from build123d import *

# Parameters (mm, degrees)
SKETCH1_W           = 25.42
SKETCH1_H           = 25.42
BOSS_EXTRUDE5_DEPTH = 4.7625
SKETCH3_W           = 4.7625
SKETCH3_H           = 61
BOSS_EXTRUDE6_DEPTH = 7.62
SKETCH4_W           = 4.7625
SKETCH4_H           = 61
BOSS_EXTRUDE7_DEPTH = 7.62
SKETCH5_W           = 76.24
SKETCH5_H           = 4.7625
BOSS_EXTRUDE8_DEPTH = 22.86


with BuildPart() as part:
    # Sketch1 → Boss-Extrude5 (new body)
    with BuildSketch(Plane.XY):
        with BuildLine():
            Line((0, 27.5), (0, 30.5))
            Line((0, 30.5), (-5.08, 30.5))
            Line((-5.08, 30.5), (-5.08, 5.08))
            Line((-5.08, 5.08), (0, 5.08))
            Line((0, 5.08), (0, 22.5))
            ThreePointArc((0, 22.5), (-2.5, 25), (0, 27.5))
        make_face()
        with BuildLine():
            Line((5.08, 30.5), (0, 30.5))
            Line((0, 30.5), (0, 27.5))
            ThreePointArc((0, 27.5), (1.767766953, 26.767766953), (2.5, 25))
            ThreePointArc((2.5, 25), (1.767766953, 23.232233047), (0, 22.5))
            Line((0, 22.5), (0, 5.08))
            Line((0, 5.08), (5.08, 5.08))
            Line((5.08, 5.08), (5.08, 30.5))
        make_face()
        with BuildLine():
            Line((30.5, 5.08), (5.08, 5.08))
            Line((5.08, 5.08), (5.08, 1.626904988))
            ThreePointArc((5.08, 1.626904988), (5.911558685, 0.995350149), (6.2272, 0))
            Line((6.2272, 0), (22.7728, 0))
            ThreePointArc((22.7728, 0), (24.5, 1.7272), (26.2272, 0))
            Line((26.2272, 0), (30.5, 0))
            Line((30.5, 0), (30.5, 5.08))
        make_face()
        with BuildLine():
            Line((22.7728, 0), (6.2272, 0))
            ThreePointArc((6.2272, 0), (5.911558685, -0.995350149), (5.08, -1.626904988))
            Line((5.08, -1.626904988), (5.08, -5.08))
            Line((5.08, -5.08), (30.5, -5.08))
            Line((30.5, -5.08), (30.5, 0))
            Line((30.5, 0), (26.2272, 0))
            ThreePointArc((26.2272, 0), (24.5, -1.7272), (22.7728, 0))
        make_face()
        with BuildLine():
            Line((2.7728, 0), (0, 0))
            Line((0, 0), (0, -5.08))
            Line((0, -5.08), (5.08, -5.08))
            Line((5.08, -5.08), (5.08, -1.626904988))
            ThreePointArc((5.08, -1.626904988), (3.504649851, -1.411558685), (2.7728, 0))
        make_face()
        with BuildLine():
            Line((0, -5.08), (0, 0))
            Line((0, 0), (-2.7728, 0))
            ThreePointArc((-2.7728, 0), (-3.504649851, -1.411558685), (-5.08, -1.626904988))
            Line((-5.08, -1.626904988), (-5.08, -5.08))
            Line((-5.08, -5.08), (0, -5.08))
        make_face()
        with BuildLine():
            Line((5.08, 1.626904988), (5.08, 5.08))
            Line((5.08, 5.08), (0, 5.08))
            Line((0, 5.08), (0, 0))
            Line((0, 0), (2.7728, 0))
            ThreePointArc((2.7728, 0), (3.504649851, 1.411558685), (5.08, 1.626904988))
        make_face()
        with BuildLine():
            Line((0, 5.08), (-5.08, 5.08))
            Line((-5.08, 5.08), (-5.08, 1.626904988))
            ThreePointArc((-5.08, 1.626904988), (-3.504649851, 1.411558685), (-2.7728, 0))
            Line((-2.7728, 0), (0, 0))
            Line((0, 0), (0, 5.08))
        make_face()
        with BuildLine():
            Line((-5.08, 1.626904988), (-5.08, 5.08))
            Line((-5.08, 5.08), (-30.5, 5.08))
            Line((-30.5, 5.08), (-30.5, 0))
            Line((-30.5, 0), (-26.2272, 0))
            ThreePointArc((-26.2272, 0), (-24.5, 1.7272), (-22.7728, 0))
            Line((-22.7728, 0), (-6.2272, 0))
            ThreePointArc((-6.2272, 0), (-5.911558685, 0.995350149), (-5.08, 1.626904988))
        make_face()
        with BuildLine():
            ThreePointArc((-5.08, -1.626904988), (-5.911558685, -0.995350149), (-6.2272, 0))
            Line((-6.2272, 0), (-22.7728, 0))
            ThreePointArc((-22.7728, 0), (-24.5, -1.7272), (-26.2272, 0))
            Line((-26.2272, 0), (-30.5, 0))
            Line((-30.5, 0), (-30.5, -5.08))
            Line((-30.5, -5.08), (-5.08, -5.08))
            Line((-5.08, -5.08), (-5.08, -1.626904988))
        make_face()
        with BuildLine():
            Line((0, -22.5), (0, -5.08))
            Line((0, -5.08), (-5.08, -5.08))
            Line((-5.08, -5.08), (-5.08, -30.5))
            Line((-5.08, -30.5), (0, -30.5))
            Line((0, -30.5), (0, -27.5))
            ThreePointArc((0, -27.5), (-2.5, -25), (0, -22.5))
        make_face()
        with BuildLine():
            Line((5.08, -5.08), (0, -5.08))
            Line((0, -5.08), (0, -22.5))
            ThreePointArc((0, -22.5), (1.767766953, -23.232233047), (2.5, -25))
            ThreePointArc((2.5, -25), (1.767766953, -26.767766953), (0, -27.5))
            Line((0, -27.5), (0, -30.5))
            Line((0, -30.5), (5.08, -30.5))
            Line((5.08, -30.5), (5.08, -5.08))
        make_face()
        with Locations((-17.79, 17.79)):
            Rectangle(SKETCH1_W, SKETCH1_H)
        with Locations((17.79, 17.79)):
            Rectangle(SKETCH1_W, SKETCH1_H)
        with Locations((17.79, -17.79)):
            Rectangle(SKETCH1_W, SKETCH1_H)
        with Locations((-17.79, -17.79)):
            Rectangle(SKETCH1_W, SKETCH1_H)
    extrude(amount=BOSS_EXTRUDE5_DEPTH)

    # Sketch3 → Boss-Extrude6 (add)
    with BuildSketch(Plane.ZY.offset(30.5)):
        with Locations((2.38125, 0)):
            Rectangle(SKETCH3_W, SKETCH3_H)
    extrude(amount=BOSS_EXTRUDE6_DEPTH)

    # Sketch4 → Boss-Extrude7 (add)
    with BuildSketch(Plane(origin=(30.5, 0, 0), x_dir=(0, 0, -1), z_dir=(1, 0, 0))):
        with Locations((-2.38125, 0)):
            Rectangle(SKETCH4_W, SKETCH4_H)
    extrude(amount=BOSS_EXTRUDE7_DEPTH)

    # Sketch5 → Boss-Extrude8 (add)
    with BuildSketch(Plane(origin=(0, 30.5, 0), x_dir=(1, 0, 0), z_dir=(0, 1, 0))):
        with Locations((0, -2.38125)):
            Rectangle(SKETCH5_W, SKETCH5_H)
    extrude(amount=BOSS_EXTRUDE8_DEPTH)


solid = part.part
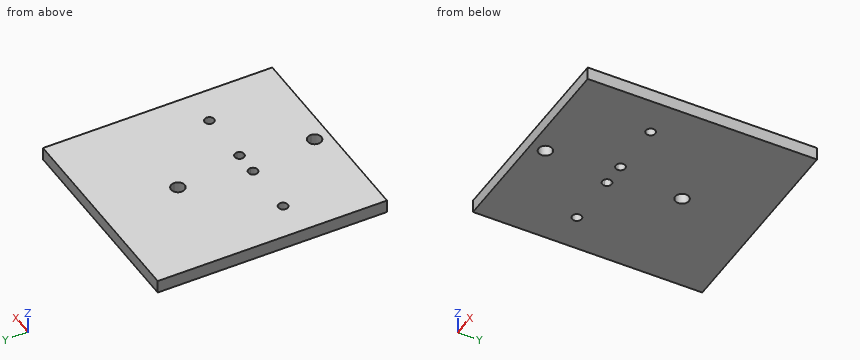
Model file for the job. Use its own axes, mm. Give positions to 0.01 mm unless a question says otherwise; leave off trailing zeros. Order: outer loops, then holes, each group sorted by start corner. A loop starts at its lowest first (then second) coordinate and runs counter-clockwise, first axis right, second up. Notation, with made-up numbers: M 43.25,-17 L 58.25,-17 A35 ccw 58.25,18 Z; hole C 54.5,46 d11. An arc over 180 degrees is marked long. Put each result on its own line as item: value. Start each with the question number.
(1) Drill centre lines: L1, parallel to Y at x = -24.5, z = 1.65; L2, parallel to X at y = -0.5, z = 4.2; L3, parallel to X at y = 23, z = 2.95. Where is each one in solid material? Low to high. Write a range as [from, to].
(2) Band-saw the part on A-A on x = 24.5. Give the cut face in (y, z), then the cut area to 3 significant figures.
(3) Pin check, flat tip, straight feed: pin 1 Ø10 at (x, y) = (15.5, 8) entering from -Z. Stop position of the tip, or through.
Results below:
1. L1: y = [-30.5, -1.73], [1.73, 53.36]
1. L2: x = [-38.12, -26.15], [-22.85, -6.15], [-2.85, 2.85], [6.15, 22.85], [26.15, 38.12]
1. L3: x = [-38.12, -1.5], [1.5, 38.12]
2. outline: M -30.5,0 L -1.73,0 L -1.73,4.76 L -30.5,4.76 Z; M 1.73,0 L 53.36,0 L 53.36,4.76 L 1.73,4.76 Z
2. area: 383 mm2
3. pin 1: stops at z = 0
